The listing builds one solid part. Answer for the finished solid, in the listing's coordinates (mm). A direction names the side the tool comes from. Round coordinates to 2 decimals unless told otherwise and drop trailing zeros. Write each loop counter-clockwise with the first axis right and the second up, starting at its lowest first coordinate (ties: lowest second). Pieces come first, ordered by that corner, then holes.
(1) A cutting plane is placed at C-C, the plane z = -18. Give the vertices of the cut face in (x, y), and give its area (3 significant figures).
(2) A cutting plane is placed at D-D, the plane x = 0. Give the vertices of the cut face in (y, z), and give its area (3 significant figures).
(3) Find the intervals of material crossed by probe 1 along X at (y, z) = (19, 18.5); probe 2 along Y at (x, z) = (39.5, 1), in increasing order.
(4) A cutting plane is placed at A-A, the plane y = 35.5. Give the vertices of the cut face in (x, z).
(5) The mould has two halves that part along Z. Classify faces 1 (the face through (-38.505, 1.232, -36.158)), 2 (the face through (-1, 17, 43)), 3 (the face through (-42, 29.61, -41.95)): +Z half, -Z half, draft (parallel to the pull), parting line (faces both ways), or undercut.
(6) A cutting plane is placed at B-B, the plane y = 17. Give the vertices of the cut face in (x, z).
(7) For faces 4 (the face through (-40.5, 29, -1)), 5 (the face through (-1, 30, 42)), 6 (the face through (34.01, 1.23, -36.16)), determine the directions among +Z, -Z, +X, -X, +Y, -Y from which every point of the face is accessible in a straight line to the end or side of a thin tool.
(8) Each of these flat-tipped pins is pushed along its axis until it touches: pin 1 Ø2.5 at (x, z) = (-36.26, 36.26) entering from +Y; pin 2 Ø3 at (x, z) = (29, -33) entering from +Y; pin 3 Ø2 at (x, z) = (-8.5, -41.5) entering from +Y. Where does it stop, or does it pass through?
from build123d import *

# Parameters (mm, degrees)
F0_W     = 81
F0_H     = 81
F0_R     = 2.25
F0_R_2   = 39
F1_DEPTH = 2.5
F0_W_2   = 86
F0_H_2   = 86
F2_DEPTH = 55
F3_W     = 81
F3_H     = 25
F4_DEPTH = 100
F5_R     = 3.5


with BuildPart() as f1:
    # F0 (on Front) → F1 (new body)
    with BuildSketch(Plane.XZ):
        Rectangle(F0_W, F0_H)
        with Locations((-36.257359, -36.257359)):
            Circle(F0_R, mode=Mode.SUBTRACT)
        with Locations((36.257359, -36.257359)):
            Circle(F0_R, mode=Mode.SUBTRACT)
        with Locations((-36.257359, 36.257359)):
            Circle(F0_R, mode=Mode.SUBTRACT)
        Circle(F0_R_2, mode=Mode.SUBTRACT)
        with Locations((36.257359, 36.257359)):
            Circle(F0_R, mode=Mode.SUBTRACT)
    extrude(amount=-F1_DEPTH)

    # F0 (on Front) → F2 (join)
    with BuildSketch(Plane.XZ):
        Rectangle(F0_W_2, F0_H_2)
        Rectangle(F0_W, F0_H, mode=Mode.SUBTRACT)
    extrude(amount=-F2_DEPTH)

    # F3 (on face) → F4 (cut)
    with BuildSketch(Plane(origin=(0, 0, -43), x_dir=(1, 0, 0), z_dir=(0, 0, -1))):
        with Locations((0, -42.5)):
            Rectangle(F3_W, F3_H)
    extrude(amount=-F4_DEPTH, mode=Mode.SUBTRACT)

    # F5
    f5_edges = [f1.edges().sort_by_distance(p)[0] for p in [
        (0, 0, -43),
        (-43, 0, 0),
        (43, 0, 0),
        (0, 0, 43),
        (-43, 27.5, 43),
        (-43, 27.5, -43),
        (43, 27.5, -43),
        (43, 27.5, 43),
    ]]
    fillet(f5_edges, radius=F5_R)


solid = f1.part
Solutions:
1. outline: (-43, 3.5) arc R3.5 ccw to (-39.5, 0) - (-34.6, 0) - (-34.6, 2.5) - (-40.5, 2.5) - (-40.5, 55) - (-43, 55) - close; (34.6, 0) - (39.5, 0) arc R3.5 ccw to (43, 3.5) - (43, 55) - (40.5, 55) - (40.5, 2.5) - (34.6, 2.5) - close
1. area: 299 mm2
2. outline: (0, -39.5) arc R3.5 ccw to (3.5, -43) - (30, -43) - (30, -40.5) - (2.5, -40.5) - (2.5, -39) - (0, -39) - close; (0, 39) - (2.5, 39) - (2.5, 40.5) - (30, 40.5) - (30, 43) - (3.5, 43) arc R3.5 ccw to (0, 39.5) - close
2. area: 152 mm2
3. probe 1: x = -43 to -40.5, 40.5 to 43
3. probe 2: y = 0 to 2.5
4. outline: (-43, -39.5) arc R3.5 ccw to (-40.5, -42.85) - (-40.5, 42.85) arc R3.5 ccw to (-43, 39.5) - close; (40.5, -42.85) arc R3.5 ccw to (43, -39.5) - (43, 39.5) arc R3.5 ccw to (40.5, 42.85) - close
5. face 1: undercut
5. face 2: +Z half
5. face 3: -Z half
6. outline: (-43, -39.5) arc R3.5 ccw to (-39.5, -43) - (39.5, -43) arc R3.5 ccw to (43, -39.5) - (43, 39.5) arc R3.5 ccw to (39.5, 43) - (-39.5, 43) arc R3.5 ccw to (-43, 39.5) - close; hole (-40.5, -40.5) - (40.5, -40.5) - (40.5, 40.5) - (-40.5, 40.5) - close
7. face 4: +Y
7. face 5: +Z, -Z, +Y
7. face 6: +Y, -Y
8. pin 1: passes through
8. pin 2: stops at y = 2.5
8. pin 3: stops at y = 30
